Can you work these out from the model? Positions are in its coordinate system, mm. A direction names the side the tool comes from. Give positions to 0.01 mm unless a question says otherwise; leave off trailing zeros. Order: outer loops, then holes, each group sorted by start corner. A loop starts at its lowest first (then second) coordinate and runs counter-clockwise, first axis right, second up. Notation, with made-up numbers: (-30, 25.25) - (26, 25.25) arc R9 ccw to (26, 37.25) - close; hole circle Ø7 at (45.25, 20). An arc over 180 degrees is marked (long way). Answer as CSV lines item,"result".
```python
from build123d import *

# Parameters (mm, degrees)
PAD_DEPTH    = 50
SKETCH002_R  = 2
PAD001_DEPTH = 4


with BuildPart() as part:
    # Sketch001 → Pad (new body)
    with BuildSketch(Plane.XY):
        with BuildLine():
            ThreePointArc((24.6079709899, -25.5870624293), (35.4957154017, 0.5515325195), (23.8011399143, 26.3392433221))
            ThreePointArc((21, 32.6458259116), (21.7317857314, 29.1954865465), (23.8011399143, 26.3392433221))
            Line((21, 32.6458259116), (21, 35.5))
            Line((21, 35.5), (0, 35.5))
            Line((0, 35.5), (0, 36.5))
            Line((0, 36.5), (21, 36.5))
            Line((21, 36.5), (22, 36.5))
            Line((22, 35.5), (22, 36.5))
            Line((22, 35.5), (22, 32.6458259714))
            ThreePointArc((22, 32.6458259714), (22.6456934726, 29.60140851), (24.4715946777, 27.0811937316))
            ThreePointArc((25.301164957, -26.3078135127), (36.4955945841, 0.5670766728), (24.4715946777, 27.0811937316))
            ThreePointArc((25.3011649571, -26.3078135128), (23.599229725, -28.7759828987), (23, -31.7135613893))
            Line((23, -31.7135613893), (23, -94.5000000518))
            ThreePointArc((22.9635179252, -94.7676438078), (22.9908375021, -94.6350594104), (23, -94.5000000518))
            Line((22.9635179252, -94.7676438078), (15.4635179477, -121.7676437268))
            Line((15.4635179477, -121.7676437268), (15.2600857185, -122.5))
            Line((14.4999999216, -122.5), (15.2600857185, -122.5))
            Line((14.4999999216, -122.5), (0, -122.5))
            Line((0, -122.5), (0, -121.5))
            Line((0, -121.5), (14.5, -121.5))
            Line((14.5, -121.5), (22, -94.5))
            Line((22, -94.5), (22, -31.7135612569))
            ThreePointArc((24.60797099, -25.5870624293), (22.6791227009, -28.3843158664), (22, -31.7135612569))
        make_face()
    pad = extrude(amount=PAD_DEPTH)

    # Sketch002 → Pad001 (join)
    with BuildSketch(Plane.XY):
        with BuildLine():
            ThreePointArc((29.2499999325, -36.5547909331), (35.2028127321, -33.411664358), (32.6312648681, -27.1905417522))
            ThreePointArc((30.5742701704, -19.9364992801), (29.9521887014, -24.0315673865), (32.6312648681, -27.1905417522))
            Line((30.5742701704, -19.9364992801), (28.638855, -21.477074))
            Line((28.638855, -21.477074), (25.3011353077, -26.3078420275))
            ThreePointArc((25.3011353077, -26.3078420275), (23.5992215491, -28.776002105), (23, -31.7135620015))
            Line((22.267235, -41.500957), (23, -31.7135620015))
            Line((23, -41.3960200869), (22.267235, -41.500957))
            ThreePointArc((29.2499999325, -36.5547909331), (24.9381378123, -37.4431730652), (23, -41.3960200869))
        make_face()
        with Locations((30.5, -31.7135617678)):
            Circle(SKETCH002_R, mode=Mode.SUBTRACT)
    pad001 = extrude(amount=PAD001_DEPTH)

    # Mirrored: Pad, Pad001 across Sketch001 V_Axis
    add(pad.mirror(Plane(origin=(0, 0, 0), x_dir=(0, 0, 1), z_dir=(1, 0, 0))))
    add(pad001.mirror(Plane(origin=(0, 0, 0), x_dir=(0, 0, 1), z_dir=(1, 0, 0))))


solid = part.part
```
1) I need wall thicknesses on line 1 along X through (y, z) = (-81.5, 41); line 2 along Y through (x, z) = (-30.5, 3.25); line 3 along Y through (x, z) = (-30, 6). Which ranges of each line are inside material? Lowest first, please. Write a range as [from, to].
Answer block:
line 1,"[-23, -22], [22, 23]"
line 2,"[-36.71, -33.71], [-29.71, -25.28], [-20.05, -18.17], [18.17, 20.05]"
line 3,"[-20.79, -18.98], [18.98, 20.79]"
2) I want a section at A-A on x = 12. Write out the boundary of the cut face in (y, z).
Answer block:
outline,"(-122.5, 0) - (-121.5, 0) - (-121.5, 50) - (-122.5, 50) - close; (35.5, 0) - (36.5, 0) - (36.5, 50) - (35.5, 50) - close"
3) I want a section at B-B on y = -43. Write out the boundary of the cut face in (x, z).
Answer block:
outline,"(-23, 0) - (-22, 0) - (-22, 50) - (-23, 50) - close; (22, 0) - (23, 0) - (23, 50) - (22, 50) - close"
4) Which directions (+Z, -Z, +X, -X, +Y, -Y) give clear straight access to the entire face, cutting with the end or side of a thin tool? Please do faces 5 (the cylindrical face through (21.71, 29.24, 24.65)), 6 (the cylindrical face through (-23.616, -28.737, 26.678)), 7 (the cylindrical face through (22.63, 29.64, 24.65)).
Answer block:
face 5,"+Z, -Z"
face 6,"+Z, -X, -Y"
face 7,"+Z, -Z, +X, +Y"
5) If we mould it in two halves opening along X, with no side actions, what happens to faces 1 (the flat face through (-23, -63, 25)), 2 (the cylindrical face through (35.5, 0.1, 24.6)), 3 (the flat face through (-28, -31, 4)), 4 (the cylindrical face through (-21.71, 29.24, 24.65))? For each: +X half, -X half, draft (parallel to the pull), parting line (faces both ways), or undercut.
Answer block:
face 1,"-X half"
face 2,"undercut"
face 3,"draft"
face 4,"undercut"
6) I'm going to push flat-ended pins straight in: P1, Ø6, axis at x = -29.5, y = -26.5, coming from the +Z side; P2, Ø2, axis at y = -47.5, z = 45, coming from the -X side; P3, Ø2.5, axis at x = -30.5, y = -31.71, coming from the -Z side; P4, Ø10, axis at x = 26.5, y = -34, coming from the +Z side. Where does each tip first touch, or does it pass through?
Answer block:
P1,"z = 4"
P2,"x = -23"
P3,"through"
P4,"z = 50"
